Build history of the part. All positions in model axes, mm. Face numbers are marked on the shaded views. A direction names the side the tool comes from. Round coordinates to 2 decimals unless told otherwise and drop trailing zeros. Order: outer loops, then holes, each group sorted by start corner. A loop starts at its lowest first (then second) coordinate and runs counter-clockwise, first axis right, second up. Notation, with made-up numbers: (89.25, 12.5) - (103.25, 12.5) arc R17 ccw to (103.25, 29.5) - close; hole circle Ø4 at (68.5, 62.25). An arc over 180 degrees is marked (long way). One line per question, with ' | ' between items. Start each with the question number.
from build123d import *

# Parameters (mm, degrees)
SKETCH1_R           = 10
SKETCH1_R_2         = 7.5
BOSS_EXTRUDE1_DEPTH = 5
SKETCH2_W           = 3
SKETCH2_H           = 15
BOSS_EXTRUDE2_DEPTH = 1


with BuildPart() as part:
    # Sketch1 → Boss-Extrude1 (new body)
    with BuildSketch(Plane(origin=(0, 0, 0), x_dir=(1, 0, 0), z_dir=(0, 1, 0))):
        with Locations(Location((0, 0, 0), (0, 0, 270))):
            Circle(SKETCH1_R)
        with Locations(Location((0, 0, 0), (0, 0, 270))):
            Circle(SKETCH1_R_2, mode=Mode.SUBTRACT)
    extrude(amount=BOSS_EXTRUDE1_DEPTH)

    # Sketch2 → Boss-Extrude2 (add)
    with BuildSketch(Plane.XZ):
        Rectangle(SKETCH2_W, SKETCH2_H)
    extrude(amount=-BOSS_EXTRUDE2_DEPTH)


solid = part.part
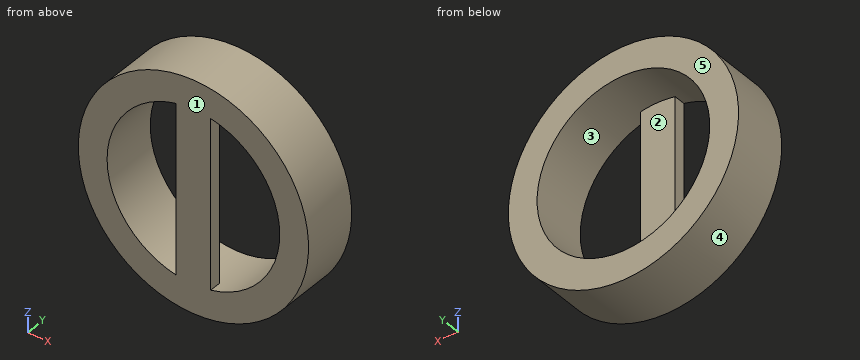
Item 1: Wall check: line 1 along X through (y, z) = (3.2, 0); line 2 along X through (y, z) = (0.55, 1.5); line 3 along Z through (x, y) = (-4.5, 4.55). Give the ranges that are in metal, low to high. Write a range as [from, to].
Item 2: Slice it at A-A (z = 0). Write the cut outline in (x, y), plus the area to 3 significant figures.
Item 3: Slice it at D-D (y = 3.2). Write the cut outline in (x, z).
Item 4: Slice it at C-C (x = 0). Write the cut outline in (y, z), plus the area to 3 significant figures.
Item 5: Pin check, flat tips, straight feed: pin 1 (1 mm diameter, centred on y = 2.5, z = 7.5, fed in from +X); pin 2 (5 mm diameter, centred on x = -7.5, z = 7.5, fed in from -Y); pin 3 (3.5 mm diameter, centred on x = -0.5, z = 2, fed in from +Y); pin 4 (0.5 mm diameter, centred on y = 0.5, z = -1, fed in from +X). Stop position of each tip, or through.
Item 6: Slice it at B-B (x = -5.5). Write the cut outline in (y, z), plus the area to 3 significant figures.
Item 7: Pull direction Z, two halves, no side cores. Call the marked faces 3, 4 and 5: released by +Z, released by -Z, zero draft, split by the parting line, or undercut.
Item 8: 3-axis set-ups, long thin cutter, end or side, ignore diameter. For the marked faces 1 and 2: which of +Z, -Z, +X, -X, +Y, -Y reach the whole face in a straight line?
A:
1) line 1: [-10, -7.5], [7.5, 10] | line 2: [-9.89, -7.35], [-1.5, 1.5], [7.35, 9.89] | line 3: [-8.93, -6], [6, 8.93]
2) outline: (-10, 0) - (-7.5, 0) - (-7.5, 5) - (-10, 5) - close; (-1.5, 0) - (1.5, 0) - (1.5, 1) - (-1.5, 1) - close; (7.5, 0) - (10, 0) - (10, 5) - (7.5, 5) - close | area: 28.0 mm^2
3) outline: circle Ø20 at (0, 0); hole circle Ø15 at (0, 0)
4) outline: (0, -10) - (5, -10) - (5, -7.5) - (1, -7.5) - (1, 7.5) - (5, 7.5) - (5, 10) - (0, 10) - close | area: 40.0 mm^2
5) pin 1: x = 7.14 | pin 2: y = 0 | pin 3: y = 1 | pin 4: x = 9.97
6) outline: (0, -8.35) - (5, -8.35) - (5, -5.1) - (0, -5.1) - close; (0, 5.1) - (5, 5.1) - (5, 8.35) - (0, 8.35) - close | area: 32.5 mm^2
7) face 3: undercut | face 4: split by the parting line | face 5: zero draft
8) face 1: +Z, -Z, +X, -X, -Y | face 2: +Y
